```python
from build123d import *

# Parameters (mm, degrees)
SKETCH_1_R      = 1.625
EXTRUDE_1_DEPTH = 3
CHAMFER_1_SIZE  = 0.5
EXTRUDE_2_DEPTH = 3


with BuildPart() as part:
    # 草图1 → 凸台-拉伸1 (new body)
    with BuildSketch(Plane(origin=(-1.5, 0, 0), x_dir=(0, -1, 0), z_dir=(-1, 0, 0))):
        with BuildLine():
            Line((4.25, -52.375771634), (4.25, 52.375771634))
            ThreePointArc((4.25, 52.375771634), (4.687412128, 55.971746395), (5.974137931, 59.357998093))
            ThreePointArc((5.974137931, 59.357998093), (0, 69.25), (-5.974137931, 59.357998093))
            ThreePointArc((-5.974137931, 59.357998093), (-4.687412128, 55.971746395), (-4.25, 52.375771634))
            Line((-4.25, 52.375771634), (-4.25, -52.375771634))
            ThreePointArc((-4.25, -52.375771634), (-4.687412128, -55.971746395), (-5.974137931, -59.357998093))
            ThreePointArc((-5.974137931, -59.357998093), (0, -69.25), (5.974137931, -59.357998093))
            ThreePointArc((5.974137931, -59.357998093), (4.687412128, -55.971746395), (4.25, -52.375771634))
        make_face()
        with Locations(Location((0, -62.5, 0), (0, 0, 270))):
            Circle(SKETCH_1_R, mode=Mode.SUBTRACT)
        with Locations(Location((0, 62.5, 0), (0, 0, 270))):
            Circle(SKETCH_1_R, mode=Mode.SUBTRACT)
    extrude(amount=-EXTRUDE_1_DEPTH)

    # 倒角1
    chamfer_1_edges = [part.edges().sort_by_distance(p)[0] for p in [
        (-1.5, -4.25, 0),
        (-1.5, -4.687412128, -55.971746395),
        (-1.5, 0, -69.25),
        (-1.5, 4.687412128, -55.971746395),
        (1.5, -4.687412128, -55.971746395),
        (1.5, -4.25, 0),
        (1.5, -4.687412128, 55.971746395),
        (1.5, 0, -60.875),
        (-1.5, 0, -60.875),
        (1.5, 0, 69.25),
        (1.5, 0, 64.125),
        (-1.5, 0, 64.125),
        (1.5, 4.687412128, 55.971746395),
        (1.5, 4.25, 0),
        (1.5, 4.687412128, -55.971746395),
        (-1.5, 4.25, 0),
        (1.5, 0, -69.25),
        (-1.5, 4.687412128, 55.971746395),
        (-1.5, 0, 69.25),
        (-1.5, -4.687412128, 55.971746395),
    ]]
    chamfer(chamfer_1_edges, length=CHAMFER_1_SIZE)

    # Sketch 3D_1 → 凸台-拉伸2 (add)
    with BuildSketch(Plane(origin=(-1.5, 1.411337563, 55.448843226), x_dir=(0, -0.022148278790467303, -0.9997546967864767), z_dir=(1, 0, 0))):
        Polygon((0, 0), (110.093393882, 2.43897747), (110.147426289, 0), (0.054032407, -2.43897747), align=None)
    extrude(amount=EXTRUDE_2_DEPTH)


solid = part.part
```
Input: part model. Units: mm. Frame: model coordinates. Give positions to 0.01 mm unless a question says otherwise; leave off trailing zeros. Order: outer loops, then holes, each group sorted by start corner. A loop starts at its lowest first (then second) coordinate and runs counter-clockwise, first axis right, second up.
1. Material intervals for L1, parallel to Y at x = 0.35, z = 62.5 (3 decimals); L2, parallel to Y at x = 1, z = -28, sorted ascending.
Derived:
L1: y = -6.75 to -1.625, 1.625 to 6.75
L2: y = -4.25 to 4.25
2. Section A-A on z = 62.5. Return the cut outline in (x, y) (3 decimals), and give its area (4 significant figures).
Derived:
outline: (-1.5, -6.25) - (-1, -6.75) - (1, -6.75) - (1.5, -6.25) - (1.5, -2.125) - (1, -1.625) - (-1, -1.625) - (-1.5, -2.125) - close; (-1.5, 2.125) - (-1, 1.625) - (1, 1.625) - (1.5, 2.125) - (1.5, 6.25) - (1, 6.75) - (-1, 6.75) - (-1.5, 6.25) - close
area: 29.75 mm2
3. Section C-C on z = 33.5. Return the cut outline in (x, y).
Derived:
outline: (-1.5, -3.75) - (-1, -4.25) - (1, -4.25) - (1.5, -3.75) - (1.5, 3.75) - (1, 4.25) - (-1, 4.25) - (-1.5, 3.75) - close
4. Mould query, pull axis Z, two halves, no side actions, for faces 1 (the cylindrical face through (-0.01, -0.49, -64.05)), 2 (the flat face through (1.5, 0, 1)). Classes: released by +Z, released by -Z, zero draft, split by the parting line, or undercut.
Derived:
face 1: undercut
face 2: zero draft
5. Section B-B on y = 0. Return the cut outline in (x, z) (3 decimals).
Derived:
outline: (-1.5, -68.75) - (-1, -69.25) - (1, -69.25) - (1.5, -68.75) - (1.5, -64.625) - (1, -64.125) - (-1, -64.125) - (-1.5, -64.625) - close; (-1.5, -60.375) - (-1, -60.875) - (1, -60.875) - (1.5, -60.375) - (1.5, 60.375) - (1, 60.875) - (-1, 60.875) - (-1.5, 60.375) - close; (-1.5, 64.625) - (-1, 64.125) - (1, 64.125) - (1.5, 64.625) - (1.5, 68.75) - (1, 69.25) - (-1, 69.25) - (-1.5, 68.75) - close
6. Pin query (flat end, axial travel): pin 1 (0.6 mm diameter, centred on x = 0, z = -25.5, fed in from +Y); pin 2 (1 mm diameter, centred on x = 0, y = -5.5, fed in from +Z); pin 3 (3.5 mm diameter, centred on y = 0, z = -62.5, fed in from -X) (3 decimals). Return the tip coordinate at first contact, or that it passes through.
Derived:
pin 1: stops at y = 4.25
pin 2: stops at z = 67.03
pin 3: stops at x = -1.125
